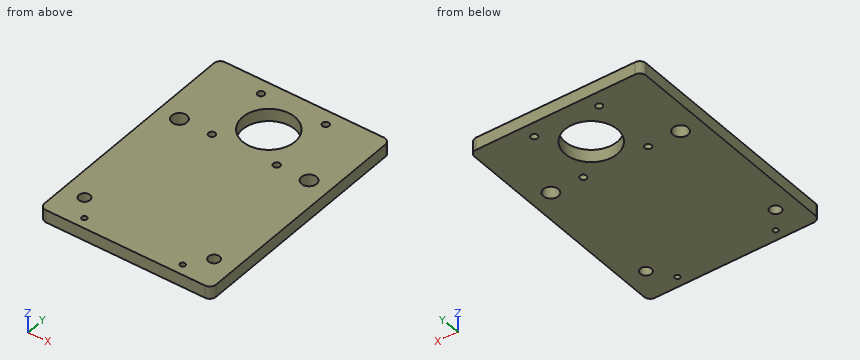
```python
from build123d import *

# Parameters (mm, degrees)
PAD010_DEPTH    = 6
SKETCH047_R     = 1.6
HOLE028_DEPTH   = 25
SKETCH050_R     = 12.5
POCKET006_DEPTH = 6.001
SKETCH048_R     = 3.6
HOLE029_DEPTH   = 25
SKETCH049_R     = 2.65
HOLE030_DEPTH   = 25
SKETCH063_R     = 1.25
HOLE032_DEPTH   = 25


with BuildPart() as part:
    # Sketch060 → Pad010 (new body)
    with BuildSketch(Plane.XY):
        with BuildLine():
            Line((-38, -8.985199), (38, -8.985199))
            ThreePointArc((41, -11.985199), (40.12132, -9.863879), (38, -8.985199))
            Line((41, -11.985199), (41, -119))
            ThreePointArc((38, -122), (40.12132, -121.12132), (41, -119))
            Line((38, -122), (-38, -122))
            ThreePointArc((-41, -119), (-40.12132, -121.12132), (-38, -122))
            Line((-41, -119), (-41, -11.985199))
            ThreePointArc((-38, -8.985199), (-40.12132, -9.863879), (-41, -11.985199))
        make_face()
    extrude(amount=PAD010_DEPTH)

    # Sketch047 (on Face10 of Pad010) → Hole028 (cut)
    with BuildSketch(Plane.XY.offset(6)):
        with Locations((-15.5, -16)):
            Circle(SKETCH047_R)
        with Locations((-15.5, -47)):
            Circle(SKETCH047_R)
        with Locations((15.5, -16)):
            Circle(SKETCH047_R)
        with Locations((15.5, -47)):
            Circle(SKETCH047_R)
    extrude(amount=-HOLE028_DEPTH, mode=Mode.SUBTRACT)

    # Sketch050 (on Face5 of Hole028) → Pocket006 (cut, through all)
    with BuildSketch(Plane.XY.offset(6)):
        with Locations((0, -31.5)):
            Circle(SKETCH050_R)
    extrude(amount=-POCKET006_DEPTH, mode=Mode.SUBTRACT)

    # Sketch048 (on Face5 of Pocket006) → Hole029 (cut)
    with BuildSketch(Plane.XY.offset(6)):
        with Locations((31, -47)):
            Circle(SKETCH048_R)
        with Locations((-31, -47)):
            Circle(SKETCH048_R)
    extrude(amount=-HOLE029_DEPTH, mode=Mode.SUBTRACT)

    # Sketch049 (on Face5 of Hole029) → Hole030 (cut)
    with BuildSketch(Plane.XY.offset(6)):
        with Locations((-31, -107)):
            Circle(SKETCH049_R)
        with Locations((31, -107)):
            Circle(SKETCH049_R)
    extrude(amount=-HOLE030_DEPTH, mode=Mode.SUBTRACT)

    # Sketch063 (on Face5 of Hole030) → Hole032 (cut)
    with BuildSketch(Plane.XY.offset(6)):
        with Locations((-23.5, -117)):
            Circle(SKETCH063_R)
        with Locations((23.5, -117)):
            Circle(SKETCH063_R)
    extrude(amount=-HOLE032_DEPTH, mode=Mode.SUBTRACT)


solid = part.part
```
The model under review builds one solid part; all positions refer to its coordinate system, in mm. Round coordinates to 2 decimals unless told otherwise and drop trailing zeros. Write each loop counter-clockwise with the first axis right and the second up, starting at its lowest first coordinate (ties: lowest second). Pieces come first, ordered by that corner, then holes. Notation, with made-up numbers: (23.25, 60) - (42.25, 60) arc R22 ccw to (42.25, 73) - close; hole circle Ø10 at (28, 68). An arc over 180 degrees is marked (long way). One line per question, with ' | ' between items.
Item 1: For P1, Ø1.9, axis at x = 15.5, y = -47, coming from the -Z side, flat-tipped, find the tip position at first contact; note if it passes through.
Resolved:
P1: passes through
Item 2: Add section D-D, the plane x = 31. Give the boundary of the cut face in (y, z), then the cut area to 3 significant figures.
Resolved:
outline: (-122, 0) - (-109.65, 0) - (-109.65, 6) - (-122, 6) - close; (-104.35, 0) - (-50.6, 0) - (-50.6, 6) - (-104.35, 6) - close; (-43.4, 0) - (-8.99, 0) - (-8.99, 6) - (-43.4, 6) - close | area: 603 mm2
Item 3: Add section B-B, the plane y = -31.5. Give the boundary of the cut face in (x, z), then the cut area to 3 significant figures.
Resolved:
outline: (-41, 0) - (-12.5, 0) - (-12.5, 6) - (-41, 6) - close; (12.5, 0) - (41, 0) - (41, 6) - (12.5, 6) - close | area: 342 mm2
Item 4: Add section C-C, the plane z = 3. State how many separate pieces and enclosed holes the cut face has, then the cut area to 3 significant figures.
Resolved:
separate pieces: 1 | enclosed holes: 11 | area: 8,600 mm2
Item 5: To check wall thickness, follow probe 1 along Y at (x, z) = (31, 2.3); probe 2 along Y at (x, z) = (-15.5, 1.95); probe 3 along X at (y, z) = (-117, 2.45). State the ranges of each line that lie inside material, in increasing order.
Resolved:
probe 1: y = -122 to -109.65, -104.35 to -50.6, -43.4 to -8.99 | probe 2: y = -122 to -48.6, -45.4 to -17.6, -14.4 to -8.99 | probe 3: x = -41 to -24.75, -22.25 to 22.25, 24.75 to 41
Item 6: Add section A-A, the plane x = 0. Give the boundary of the cut face in (y, z), then the cut area to 3 significant figures.
Resolved:
outline: (-122, 0) - (-44, 0) - (-44, 6) - (-122, 6) - close; (-19, 0) - (-8.99, 0) - (-8.99, 6) - (-19, 6) - close | area: 528 mm2
